from build123d import *

# Parameters (mm, degrees)
SKETCH1_R           = 9.525
BOSS_EXTRUDE1_DEPTH = 3.81
SKETCH2_R           = 3.006995321
BOSS_EXTRUDE2_DEPTH = 2.286
SKETCH3_R           = 0.749981853
CUT_EXTRUDE1_DEPTH  = 12.446
SKETCH4_R           = 2.02646881
CUT_EXTRUDE2_DEPTH  = 12.446


with BuildPart() as part:
    # Sketch1 → Boss-Extrude1 (new body)
    with BuildSketch(Plane(origin=(0, 0, 0), x_dir=(1, 0, 0), z_dir=(0, 1, 0))):
        with Locations(Location((0, 0, 0), (0, 0, 90))):
            Circle(SKETCH1_R)
    extrude(amount=BOSS_EXTRUDE1_DEPTH)

    # Sketch2 → Boss-Extrude2 (add)
    with BuildSketch(Plane(origin=(0, 3.81, 0), x_dir=(1, 0, 0), z_dir=(0, 1, 0))):
        with Locations(Location((0, 0, 0), (0, 0, 270))):
            Circle(SKETCH2_R)
    extrude(amount=BOSS_EXTRUDE2_DEPTH)

    # Sketch3 → Cut-Extrude1 (cut)
    with BuildSketch(Plane(origin=(0, 3.81, 0), x_dir=(1, 0, 0), z_dir=(0, 1, 0))):
        with Locations(Location((-0.749981853, 6.378803081, 0), (0, 0, 270))):
            Circle(SKETCH3_R)
        with Locations(Location((6.378803081, 0.749981853, 0), (0, 0, 270))):
            Circle(SKETCH3_R)
        with Locations(Location((0.749981853, -6.378803081, 0), (0, 0, 270))):
            Circle(SKETCH3_R)
        with Locations(Location((-6.378803081, -0.749981853, 0), (0, 0, 270))):
            Circle(SKETCH3_R)
    extrude(amount=-CUT_EXTRUDE1_DEPTH, mode=Mode.SUBTRACT)

    # Sketch4 → Cut-Extrude2 (cut)
    with BuildSketch(Plane(origin=(0, 6.096, 0), x_dir=(1, 0, 0), z_dir=(0, 1, 0))):
        with Locations(Location((0, 0, 0), (0, 0, 270))):
            Circle(SKETCH4_R)
    extrude(amount=-CUT_EXTRUDE2_DEPTH, mode=Mode.SUBTRACT)


solid = part.part
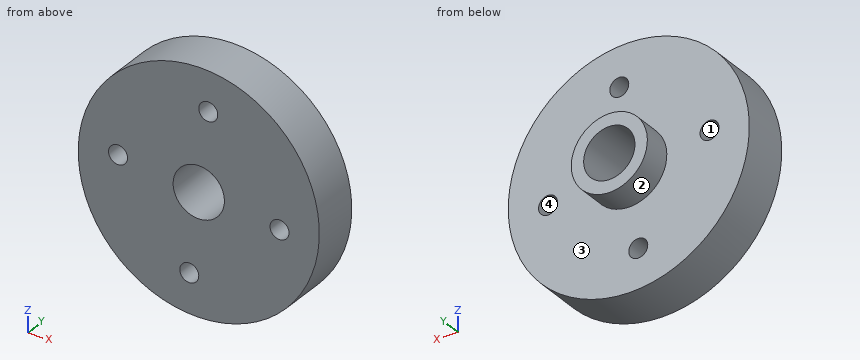
Input: part model. Units: mm. Frame: model coordinates. Face numbers are marked on the shaded views. Coordinates: 2 decimals unless noted, no trailing zeros. Loops run counter-clockwise (first coordinate to the right, second up) from the corner with the lowest first, then second, coordinate; pieces in that order, holes last. Notation, with made-up numbers: (14.5, -33) - (71.5, -33) arc R27 ccw to (71.5, -3) - close; hole circle Ø6 at (6.25, -22). An arc over 180 degrees is marked (long way). Answer in a Markdown table with one row per item. Add a question column.
Item 1: Section query D-D on x = -2.75. Return the cut outline in (y, z).
Item 2: Section query A-A on x = 1.75. Return the cut outline in (y, z).
Item 3: Section query C-C on z = 2.5. Return the cut outline in (x, y).
Item 4: Mould query, pull axis Z, two halves, no side actions, for the marked faces 1, 2, 3 and 4. Classes: released by +Z, released by -Z, zero draft, split by the parting line, or undercut.
Item 5: Contact query for flat-ended pins moving along their axis: P1, Ø3, axis at x = -5, y = 4, coming from the -Z side; P2, Ø1, axis at y = 2, z = -7, coming from the +X side; P3, Ø1.5, axis at x = -1, y = 2, coming from the +Z side; P4, Ø5.5, axis at x = 0, z = 0, coming from the -Y side. Output: stop coordinate, or through.
Item 6: Line query: line 1 along Z through (x, y) = (-0.75, 1.75); line 2 along Y through (x, z) = (1.5, -3.5); line 3 along X through (y, z) = (2.5, -1.25). Output: solid intervals per line, ascending. Write a range as [from, to].
Item 7: Section query B-B on y = 1.25. Return the cut outline in (x, z) (3 decimals).
Recorded:
| question | item | result |
|---|---|---|
| 1 | outline | (0, -9.12) - (3.81, -9.12) - (3.81, -1.22) - (6.1, -1.22) - (6.1, 1.22) - (3.81, 1.22) - (3.81, 9.12) - (0, 9.12) - close |
| 2 | outline | (0, -9.36) - (3.81, -9.36) - (3.81, -2.45) - (6.1, -2.45) - (6.1, -1.02) - (0, -1.02) - close; (0, 1.02) - (6.1, 1.02) - (6.1, 2.45) - (3.81, 2.45) - (3.81, 9.36) - (0, 9.36) - close |
| 3 | outline | (-9.19, 0) - (9.19, 0) - (9.19, 3.81) - (1.67, 3.81) - (1.67, 6.1) - (-1.67, 6.1) - (-1.67, 3.81) - (-9.19, 3.81) - close |
| 4 | face 1 | undercut |
| 4 | face 2 | split by the parting line |
| 4 | face 3 | zero draft |
| 4 | face 4 | undercut |
| 5 | P1 | z = -8.85 |
| 5 | P2 | x = 6.96 |
| 5 | P3 | z = 9.52 |
| 5 | P4 | y = 0 |
| 6 | line 1 | [-9.5, -7.13], [-5.63, -1.88], [1.88, 9.5] |
| 6 | line 2 | [0, 3.81] |
| 6 | line 3 | [-9.44, -1.6], [1.6, 5.82], [6.94, 9.44] |
| 7 | outline | circle Ø19.05 at (0, 0); hole circle Ø1.5 at (-6.379, 0.75); hole circle Ø4.053 at (0, 0); hole circle Ø1.5 at (-0.75, -6.379); hole circle Ø1.5 at (0.75, 6.379); hole circle Ø1.5 at (6.379, -0.75) |
